Study the drawing (mm; zero at the part's minimum x, y, z) and answer. A direction names the side the tool comes from. Coordinates: 2 decimals unless noted, no trailing zeros. Order: outer loops, then holes, each group sorted by start corner. A loop starts at its lowest first (then second) coordinate and runs counter-clockwise, first axis right, second up. Notation, with made-up numbers: M 70.5,85.25 L 84.5,85.25 A14 cw 84.5,107.25 Z; hole C 87,19 d10. An arc over 180 degrees is marked long. Put each result on its own line as item: value.
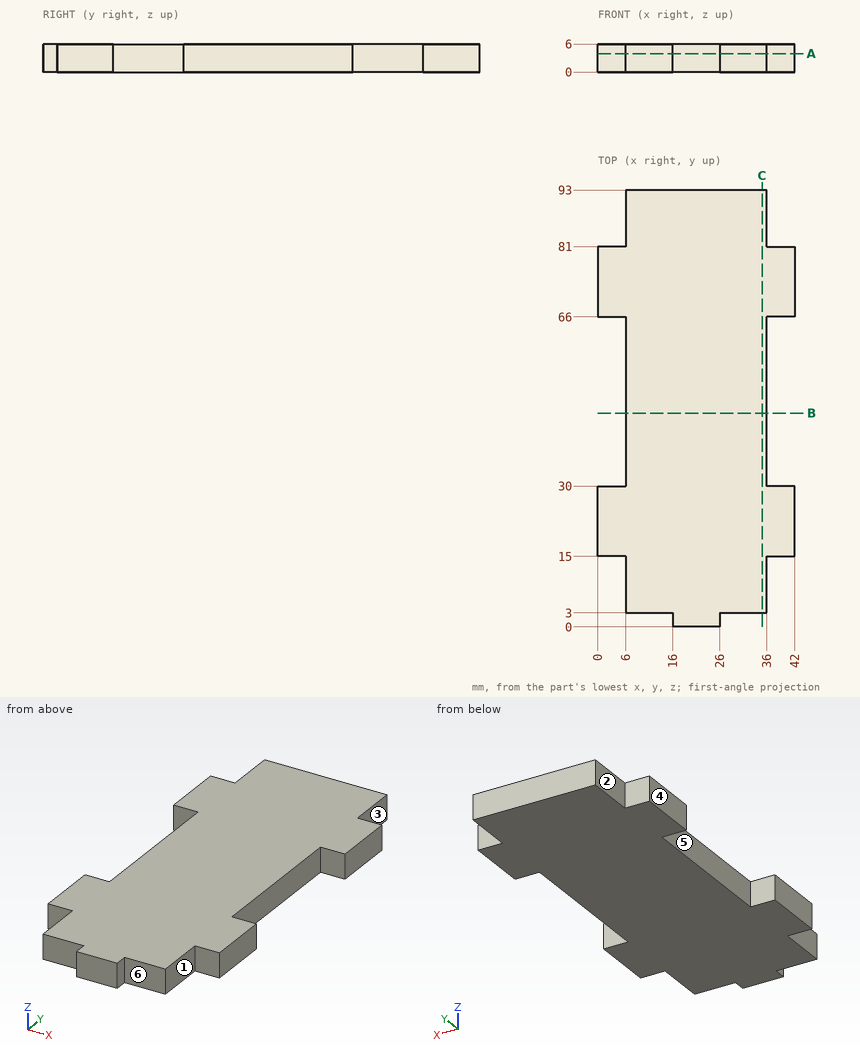
Q1. Find section C-C on x = 35. Write down the section's boundary in (y, z).
Answers below:
outline: M 3,0 L 93,0 L 93,6 L 3,6 Z
Q2. Find section A-A on z = 3.95. Write down the section's boundary in (x, y).
Answers below:
outline: M 0,15 L 6,15 L 6,3 L 16,3 L 16,0 L 26,0 L 26,3 L 36,3 L 36,15 L 42,15 L 42,30 L 36,30 L 36,66 L 42,66 L 42,81 L 36,81 L 36,93 L 6,93 L 6,81 L 0,81 L 0,66 L 6,66 L 6,30 L 0,30 Z
Q3. Find section B-B on y = 45.5. Write down the section's boundary in (x, z), plus the area to 3 significant figures.
Answers below:
outline: M 6,0 L 36,0 L 36,6 L 6,6 Z
area: 180 mm^2
Q4. A tool of negligible diameter and unlimited length cuts with its end or side. For the marked faces 1, 2 and 3, from which of +Z, -Z, +X, -X, +Y, -Y can it reach the whole face along a straight path? Write none if from no direction.
Answers below:
face 1: +Z, -Z, +X, -Y
face 2: +Z, -Z, -X, +Y
face 3: +Z, -Z, +X, +Y
Q5. Given pin 1 (1.8 mm diameter, centred on x = 39, z = 2.5, fed in from -Y); pin 2 (0.9 mm diameter, centred on y = 1, z = 3, fed in from -X); pin 3 (2.5 mm diameter, centred on y = 1.5, z = 3.5, fed in from +X), each flat-ended and moving along its own axis, determine where each tip first touches the part or whether it passes through.
Answers below:
pin 1: stops at y = 15
pin 2: stops at x = 16
pin 3: stops at x = 26
Q6. Consider line 1 along Y through (x, z) = (37, 3.7); line 2 along X through (y, z) = (8.5, 1.55); line 3 along Y through (x, z) = (32.5, 4.9). Determine where each line is inside the solid, lowest interval first.
Answers below:
line 1: y = 15 to 30, 66 to 81
line 2: x = 6 to 36
line 3: y = 3 to 93
Q7. For a pull along Y with two mould halves and no side action, classify the marked faces 4, 5 and 6 as +Y half, -Y half, draft (parallel to the pull), parting line (faces both ways), or undercut.
Answers below:
face 4: draft
face 5: undercut
face 6: -Y half
